Verification items for the finished model (mm, model axes). A direction names the side the tool comes from. Coordinates: 2 decimals unless noted, no trailing zeros. Order: outer loops, then holes, each group sorted by start corner. A loop starts at its lowest first (then second) coordinate and runs counter-clockwise, first axis right, second up. Notation, with made-up numbers: M 35.5,12 L 91.5,12 A25 cw 91.5,48 Z; hole C 44,78 d6. An arc over 180 degrees is marked long. Return JSON: item names as keys, results as strings. Group by question number.
1. Section check C-C, the plane x = -0.8. Record the cut outline in (y, z), plus the area to 3 significant figures.
2. Gauge pin test, flat ends, axial feed: pin 1 (4 mm diameter, centred on y = 4.5, z = -5.5, fed in from -X); pin 2 (1 mm diameter, centred on x = -1.5, y = 6, fed in from -Z); pin 3 (1.3 mm diameter, centred on x = -1, y = 4, fed in from -Z). Record the tip position at first contact, or that the pin passes through.
3. Section check B-B, the plane y = 6.35. Record the cut outline in (x, z), plus the area to 3 significant figures.
4. Material ranges on line 1 along Y through (x, z) = (-0.8, -3.81); line 2 along X through (y, z) = (8.75, -2.25); line 3 along Y through (x, z) = (-1, -3.25), recorded low to high.
5. Mould release check, pull along Y, two halves, no side actions. Record for faces 1 (the flat face through (-1, 5, -6.426)), 2 (the cylindrical face through (-1.25, 7.02, -3.08)), 3 (the flat face through (-3, 0.254, -4)): +Y half, -Y half, draft (parallel to the pull), parting line (faces both ways), or undercut.
6. Section check A-A, the plane z = -3.81. Record the cut outline in (x, y), plus the area to 3 significant figures.
7. Section check D-D, the plane y = 2.25. Record the cut outline in (x, z).
8. Set-up check for faces 4 (the flat face through (-2, 0, -4)), 5 (the flat face through (-1, 5, -1.194)), 6 (the flat face through (-2.533, 5, -4)): record each of +Z, -Z, +X, -X, +Y, -Y from which the full face is reachable in a straight line by a thin tool's end or side.
Autodesk Inventor part; units mm, degrees
ref_plane "YZ Plane" through (0, 0, 0) normal (1, 0, 0) x (0, 1, 0)
ref_plane "XZ Plane" through (0, 0, 0) normal (0, 1, 0) x (-1, 0, 0)
ref_plane "XY Plane" through (0, 0, 0) normal (0, 0, 1) x (1, 0, 0)
sketch "Sketch1" plane through (0, 0, 0) normal (0, 1, 0) x (-1, 0, 0)
  line L0 (0, -6.4262) -> (0, -1.1938)
  arc A0 (1.1938, -1.1938) -> (2.3876, 0) centre (1.1938, 0) ccw
  arc A1 (2.3876, -7.62) -> (1.1938, -6.4262) centre (1.1938, -7.62) ccw
  line L1 (2.3876, 0) -> (2.5329, 0)
  line L2 (2.5329, 0) -> (2.5329, -7.62)
  line L3 (2.5329, -7.62) -> (2.3876, -7.62)
  line L4 (1.1938, -6.4262) -> (0, -6.4262)
  line L5 (1.1938, -1.1938) -> (0, -1.1938)
  line L6 (0, 0) -> (3.3528, 0)
  line L7 (0, -3.81) -> (2.5329, -3.81)
  line L8 (0, -7.62) -> (3.3528, -7.62)
  line L9 (3.3528, -7.62) -> (3.3528, 0)
  dimension "d2" = 2.3876
  dimension "d3" = 2.3876
  dimension "d12" = 3.3528
extrude "Extrusion1" add sketch "Sketch1" along normal blind 10.16 contours L0 L7 L2 L3 A1 L4 | L0 L5 A0 L1 L2 L7
sketch "Sketch2" plane through (0, 0, -1.1938) normal (1, 0, 0) x (0, 0, -1)
  circle A0 centre (2.6162, 6.35) radius 0.9922
  line L0 (0, 0) -> (5.2324, 0)
  point P0 (-1.1938, 0)
  dimension "d8" = 1.9844
  dimension "d9" = 6.35
extrude "Extrusion3" cut sketch "Sketch2" against normal blind 127
extrude "Extrusion4" add sketch "Sketch1" along normal blind 0.254 contours L2 L6 L9 L8
properties part number "Ease of Model Bearing"
Answers follow:
{
 "1": {"outline": "M 0,-6.43 L 10.16,-6.43 L 10.16,-1.19 L 0,-1.19 Z; hole C 6.35,-3.81 d1.98", "area": "50.1 mm^2"},
 "2": {"pin 1": "x = -2.53", "pin 2": "z = -6.74", "pin 3": "z = -6.52"},
 "3": {"outline": "M -2.53,-7.62 L -2.39,-7.62 A1.19 cw -1.19,-6.43 L 0,-6.43 L 0,-4.8 L -2.53,-4.8 Z; M -2.53,-2.82 L 0,-2.82 L 0,-1.19 L -1.19,-1.19 A1.19 cw -2.39,0 L -2.53,0 Z", "area": "9.19 mm^2"},
 "4": {"line 1": "0 to 5.36, 7.34 to 10.16", "line 2": "-2.53 to 0", "line 3": "0 to 5.53, 7.17 to 10.16"},
 "5": {"face 1": "draft", "face 2": "undercut", "face 3": "+Y half"},
 "6": {"outline": "M -3.35,0 L 0,0 L 0,5.36 L -2.53,5.36 L -2.53,0.25 L -3.35,0.25 Z; M -2.53,7.34 L 0,7.34 L 0,10.16 L -2.53,10.16 Z", "area": "20.9 mm^2"},
 "7": {"outline": "M -2.53,-7.62 L -2.39,-7.62 A1.19 cw -1.19,-6.43 L 0,-6.43 L 0,-1.19 L -1.19,-1.19 A1.19 cw -2.39,0 L -2.53,0 Z"},
 "8": {"face 4": "+Z, -Z, +X, -X, -Y", "face 5": "+Z, +X, +Y, -Y", "face 6": "+Z, -Z, -X, +Y"}
}
